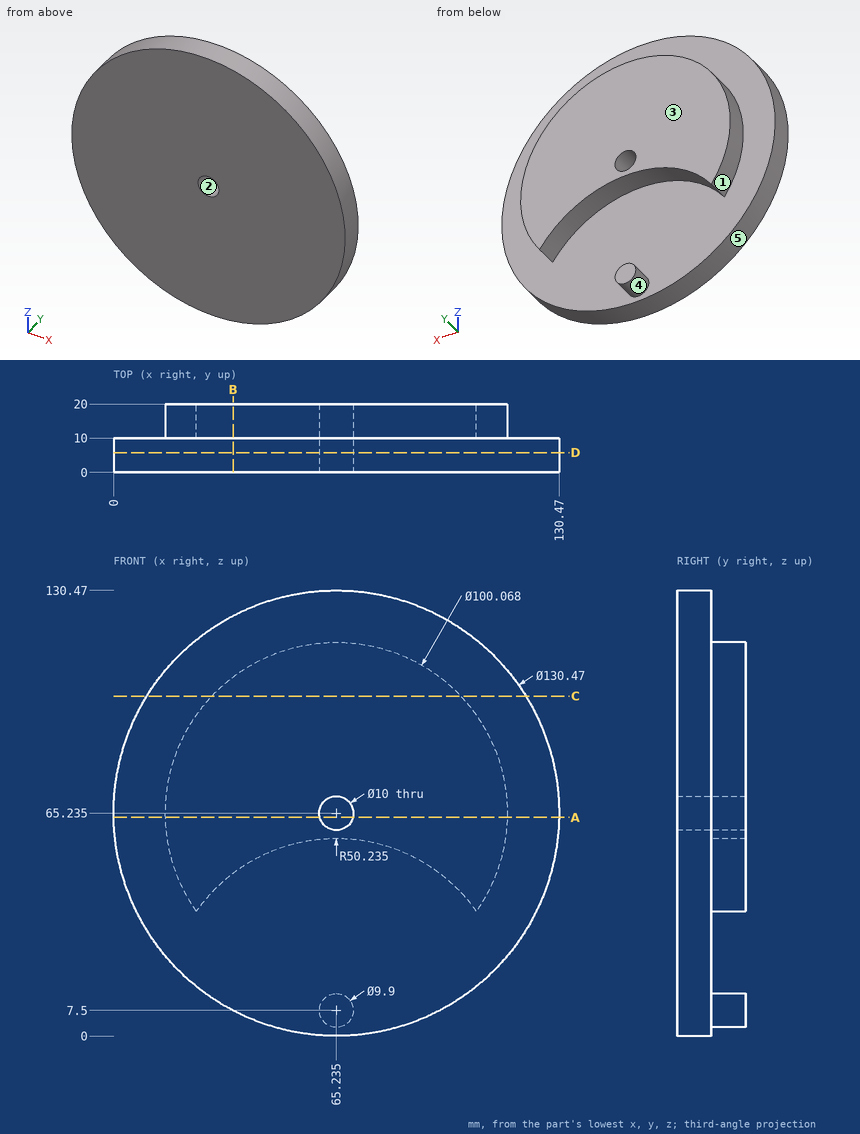
Could you check a few things on this drawing? It's one solid part, dimensions in mm from its lowest x, y, z. A direction names the side the tool comes from. Coordinates: 2 decimals unless noted, no trailing zeros. Write each loop counter-clockwise with the first axis right and the second up, starting at its lowest first coordinate (ties: lowest second). Pieces come first, ordered by that corner, then holes. Notation, with made-up numbers: (52.5, 14) - (86.5, 14) arc R21 cw to (86.5, 35) - close; hole circle Ø10 at (3.5, 69.25). An arc over 180 degrees is marked (long way). Put each result on its own line as item: value. Start each with the question number.
Q1. Thinking about a two-plate mould opening in X: for the marked faces 1, 2 and 3, which applies, pulls with the +X half, pulls with the -X half, needs draft (parallel to the pull), parting line crosses it, or undercut?
Q2. I want a section at B-B on x = 35. Write out the boundary of the cut face in (y, z), plus the area to 3 significant figures.
Q3. I want a section at A-A on z = 64. Write out the boundary of the cut face in (x, y), plus the area to 3 significant figures.
Q4. Which directions (+Z, -Z, +X, -X, +Y, -Y) give clear straight access to the entire face, cutting with the end or side of a thin tool? Please do the marked faces 4 and 5.
Q5. I want a section at C-C on z = 99.5. Write out the boundary of the cut face in (x, y) (1 decimal).
Q6. I want a section at D-D on y = 5.75. Write out the boundary of the cut face in (x, z) (1 decimal), plus the area to 3 significant figures.
Q7. Please list where these lines run through material, in increasing order: L1, parallel to Z at x = 62, y = 16.25 (1 decimal); L2, parallel to Y at x = 103.5, z = 22.5; L3, parallel to X at y = 15, z = 40.5.
Q8. I'm going to push flat-ended pins straight in: P1, Ø13, axis at x = 65.24, z = 65.24, coming from the -Y side; P2, Ø1.5, axis at x = 60, y = 6, coming from the -Z side; P3, Ø4, axis at y = 2.5, z = 32, coming from the +X side; P4, Ø10, axis at y = 14, z = 22, coming from the -X side (1 decimal). Where does each tip first touch, or does it pass through?
Checks:
1. face 1: parting line crosses it
1. face 2: undercut
1. face 3: needs draft
2. outline: (0, 7.43) - (10, 7.43) - (10, 47.62) - (20, 47.62) - (20, 105.1) - (10, 105.1) - (10, 123.04) - (0, 123.04) - close
2. area: 1,730 mm²
3. outline: (0.01, 0) - (60.39, 0) - (60.39, 20) - (15.22, 20) - (15.22, 10) - (0.01, 10) - close; (70.08, 0) - (130.46, 0) - (130.46, 10) - (115.25, 10) - (115.25, 20) - (70.08, 20) - close
3. area: 2,110 mm²
4. face 4: +Y
4. face 5: +Y, -Y
5. outline: (9.7, 0) - (120.7, 0) - (120.7, 10) - (101.7, 10) - (101.7, 20) - (28.8, 20) - (28.8, 10) - (9.7, 10) - close
6. outline: circle Ø130.5 at (65.2, 65.2); hole circle Ø10 at (65.2, 65.2)
6. area: 13,300 mm²
7. L1: 3.8 to 11.2, 57.6 to 61.4, 69 to 115.2
7. L2: 0 to 10
7. L3: 21.74 to 27.36, 103.11 to 108.73
8. P1: y = 0
8. P2: z = 0.15
8. P3: x = 122.51
8. P4: x = 13.9
